Build history of the part. All positions in model axes, mm. A direction names the side the tool comes from. Coordinates: 2 decimals unless noted, no trailing zeros. Order: outer loops, then holes, each group sorted by start corner. A loop starts at its lowest first (then second) coordinate and runs counter-clockwise, first axis right, second up. Notation, with made-up numbers: (44.5, 53) - (95.5, 53) arc R23 ccw to (95.5, 75) - close; hole circle Ø11 at (10, -24). An arc over 180 degrees is marked (long way). Answer as CSV lines item,"result". Start each with the question number.
from build123d import *

# Parameters (mm, degrees)
BOSS_EXTRUDE1_DEPTH             = 2
FILLET1_R                       = 4
CUT_EXTRUDE1_REACH              = 137.809
SKETCH2_R                       = 1.55
BOSS_EXTRUDE2_DEPTH             = 12
BOSS_EXTRUDE2_DIRECTION_2_REACH = 137.809
BOSS_EXTRUDE3_DEPTH             = 20
FILLET2_R                       = 4
CUT_EXTRUDE2_REACH              = 70.911
SKETCH5_R                       = 1.55


with BuildPart() as part:
    # Sketch1 → Boss-Extrude1 (new body)
    with BuildSketch(Plane.XY):
        Polygon((70, 114.805547545), (60.427350908, 97.245240333), (53.403228024, 101.07429997), (62.975877115, 118.634607181), align=None)
    extrude(amount=BOSS_EXTRUDE1_DEPTH)

    # Fillet1
    fillet1_edges = [part.edges().sort_by_distance(p)[0] for p in [
        (60.427350908, 97.245240333, 1),
        (53.403228024, 101.07429997, 1),
        (70, 114.805547545, 1),
        (62.975877115, 118.634607181, 1),
    ]]
    fillet(fillet1_edges, radius=FILLET1_R - 0.0001)  # a hair under: the kernel refuses the full size

    # Sketch2 → Cut-Extrude1 (cut, up to next)
    with BuildSketch(Plane.XY.offset(2), mode=Mode.PRIVATE) as cut_extrude1_sk1:
        with Locations((64.573408739, 113.208015921)):
            Circle(SKETCH2_R)
    cut_extrude1_tool1 = extrude(cut_extrude1_sk1.sketch, amount=-CUT_EXTRUDE1_REACH, mode=Mode.PRIVATE) & part.part
    # Sketch2 → Cut-Extrude1 (cut, up to next)
    with BuildSketch(Plane.XY.offset(2), mode=Mode.PRIVATE) as cut_extrude1_sk2:
        with Locations((58.829819284, 102.671831594)):
            Circle(SKETCH2_R)
    cut_extrude1_tool2 = extrude(cut_extrude1_sk2.sketch, amount=-CUT_EXTRUDE1_REACH, mode=Mode.PRIVATE) & part.part
    add(cut_extrude1_tool1.solids().sort_by_distance((64.573409, 113.208016, 2))[0], mode=Mode.SUBTRACT)
    add(cut_extrude1_tool2.solids().sort_by_distance((58.829819, 102.671832, 2))[0], mode=Mode.SUBTRACT)

    # Sketch3 → Boss-Extrude2 (add)
    with BuildSketch(Plane.XY.offset(2)):
        Polygon((66.170940363, 107.78142466), (59.146817479, 111.610484297), (53.878725315, 114.482279024), (51.964195497, 110.970217582), (57.23228766, 108.098422855), (64.256410545, 104.269363218), (69.524502708, 101.39756849), (71.439032527, 104.909629933), align=None)
    extrude(amount=BOSS_EXTRUDE2_DEPTH)

    # Boss-Extrude2 direction 2: up to this face of the body (flat: up to its plane)
    boss_extrude2_direction_2_end = Plane(part.part.faces().sort_by_distance((61.701614012, 107.939923757, 0))[0])
    # Sketch3 → Boss-Extrude2 direction 2 (add, up to the picked face)
    with BuildSketch(Plane.XY.offset(2), mode=Mode.PRIVATE) as boss_extrude2_direction_2_sk1:
        Polygon((66.170940363, 107.78142466), (59.146817479, 111.610484297), (53.878725315, 114.482279024), (51.964195497, 110.970217582), (57.23228766, 108.098422855), (64.256410545, 104.269363218), (69.524502708, 101.39756849), (71.439032527, 104.909629933), align=None)
    boss_extrude2_direction_2_tool1 = split(extrude(boss_extrude2_direction_2_sk1.sketch, amount=-BOSS_EXTRUDE2_DIRECTION_2_REACH, mode=Mode.PRIVATE), bisect_by=boss_extrude2_direction_2_end, keep=Keep.BOTH, mode=Mode.PRIVATE)
    add(boss_extrude2_direction_2_tool1.solids().sort_by(Axis((61.701614, 107.939924, 2), (0, 0, -1)))[0])

    # Sketch4 → Boss-Extrude3 (add)
    with BuildSketch(Plane(origin=(-6.575093345, 3.584280194, 0), x_dir=(0, 0, 1), z_dir=(-0.8780153605811593, 0.4786324545865408, 0))):
        Polygon((22.660254038, 121.305306045), (20.92820323, 118.305306045), (14, 122.305306045), (14, 126.305306045), align=None)
    extrude(amount=-BOSS_EXTRUDE3_DEPTH)

    # Fillet2
    fillet2_edges = [part.edges().sort_by_distance(p)[0] for p in [
        (50.76761436, 108.775179181, 21.794228634),
        (68.327921572, 99.202530089, 21.794228634),
    ]]
    fillet(fillet2_edges, radius=FILLET2_R)

    # Sketch5 → Cut-Extrude2 (cut, up to next)
    with BuildSketch(Plane(origin=(48.241919048, 88.496184373, 58.191801834), x_dir=(0.9100457296544759, -0.34633972242186517, -0.22774012955647066), z_dir=(0.41450786474764584, 0.7603836071762374, 0.5000000000000009)), mode=Mode.PRIVATE) as cut_extrude2_sk1:
        with Locations(Location((8.475365681, 44.360860805, 0), (0, 0, 270))):
            Circle(SKETCH5_R)
    cut_extrude2_tool1 = extrude(cut_extrude2_sk1.sketch, amount=-CUT_EXTRUDE2_REACH, mode=Mode.PRIVATE) & part.part
    # Sketch5 → Cut-Extrude2 (cut, up to next)
    with BuildSketch(Plane(origin=(48.241919048, 88.496184373, 58.191801834), x_dir=(0.9100457296544759, -0.34633972242186517, -0.22774012955647066), z_dir=(0.41450786474764584, 0.7603836071762374, 0.5000000000000009)), mode=Mode.PRIVATE) as cut_extrude2_sk2:
        with Locations(Location((20.053008413, 41.205201002, 0), (0, 0, 270))):
            Circle(SKETCH5_R)
    cut_extrude2_tool2 = extrude(cut_extrude2_sk2.sketch, amount=-CUT_EXTRUDE2_REACH, mode=Mode.PRIVATE) & part.part
    add(cut_extrude2_tool1.solids().sort_by_distance((55.954889, 109.933703, 19.196152))[0], mode=Mode.SUBTRACT)
    add(cut_extrude2_tool2.solids().sort_by_distance((66.491074, 104.190114, 19.196152))[0], mode=Mode.SUBTRACT)


solid = part.part
(1) Drop flat-ended pins along their axis: pin 1 Ø10.5 at (x, y) = (63, 112.5) entering from +Z; pin 2 Ø3 at (x, y) = (58.83, 102.67) entering from -Z; pin 3 Ø1.5 at (y, z) = (109.5, 6.5) entering from -X. Give the stop position or say it passes through.
(2) Band-saw the part on D-D on z = 1.5. State how many separate pieces and enclosed holes the cut face has, plus the area to 3 significant figures.
(3) Band-saw the part on A-A on y = 113.5. List the corners of the cut face in (x, z).
(4) Band-saw the part on C-C on x = 57.75. List the corners of the cut face in (y, z), plus the area to 3 significant figures.
(5) Pull direction X, two halves, no side cores. Call faces 1 (the flat face through (67.14, 109.56, 0.99)), 2 (the flat face through (62, 108, 0)), 3 (the flat face through (63.313, 102.538, 0.986)), 4 (the flat face through (56.262, 106.318, 0.986)): +X half, -X half, draft (parallel to the pull), parting line (faces both ways), or undercut.
(6) Probe L1, parallel to Z at x = 67.5, y = 115; L2, parallel to X at y = 111, z = 12.5; L3, parallel to Y at x = 69, z = 15.25. List the from-to ranges inside material, lowest first. Write a range as [from, to].
(7) Which spindle directions (+Z, -Z, +X, -X, +Y, -Y) get a long thin tool onto all of the face, cutting with end or side? Do faces 5 (the flat face through (60.09, 113.34, 0.99)), 6 (the cylindrical face through (59.55, 101.3, 1.01)), 7 (the flat face through (63.9, 111.5, 2)). Say none if no direction does.
(8) Band-saw the part on B-B on z = 8.25. List the corners of the cut face in (x, y), plus the area to 3 significant figures.
Filled in:
1,pin 1,"stops at z = 18.55"
1,pin 2,"stops at z = 18.33"
1,pin 3,"stops at x = 53.29"
2,separate pieces,"1"
2,enclosed holes,"2"
2,area,"179 mm^2"
3,outline,"(53.34, 0) - (55.68, 0) - (55.68, 14) - (53.34, 15.94) - close; (60.18, 0) - (63.05, 0) - (63.05, 2) - (60.18, 2) - close; (66.1, 0) - (68.56, 0) - (68.56, 2) - (66.1, 2) - close"
4,outline,"(98.82, 0) - (101.56, 0) - (101.56, 2) - (98.82, 2) - close; (103.26, 20.93) - (107.82, 14) - (107.82, 2) - (103.78, 2) - (103.78, 0) - (112.37, 0) - (112.37, 14) - (106.68, 22.66) - close"
4,area,"113 mm^2"
5,face 1,"+X half"
5,face 2,"draft"
5,face 3,"undercut"
5,face 4,"-X half"
6,L1,"z = [0, 2]"
6,L2,"x = [51.98, 60.27]"
6,L3,"y = [100.86, 105.42]"
7,face 5,"+Z, -Z, +Y"
7,face 6,"-Z"
7,face 7,"+Z, +X, +Y"
8,outline,"(51.96, 110.97) - (69.52, 101.4) - (71.44, 104.91) - (53.88, 114.48) - close"
8,area,"80.0 mm^2"
